Geometry check sheet. Reference: drawing and pictorial views, mm from the part's lowest x, y, z. A direction names the side the tool comes from. Round coordinates to 2 decimals unless told otherwise and drop trailing zeros. Loops run counter-clockwise (first coordinate to the right, second up) from the corner with the lowest first, then second, coordinate; pieces in that order, holes last. Notation, with made-up numbers: M -9,-7 L 40,-7 A9 cw 40,-1 Z; hole C 41.25,-34.75 d9. An arc over 180 degrees is marked long. One line per question, with ' | ' between items. Start each with the question number.
(1) Section check C-C (x = 2.25). Record the boundary of the cut face in (y, z) (1 decimal).
(2) Draft check along Z on the marked faces 1, 2 and 3. Enter one of: +Z half, -Z half, draft (parallel to the pull), parting line (faces both ways), or undercut.
(3) Section check B-B (z = 2.7). Record the boundary of the cut face in (x, y).
(4) Thickness scan on probe 1 along Z at (x, y) = (2.6, 3); probe 2 along Y at (x, z) = (4.6, 4.2); probe 3 along Y at (x, z) = (3.7, 3.35). Record the ranges inside material, lowest first. Write a range as [from, to].
(5) Section check D-D (y = 3.75). Record the boundary of the cut face in (x, z).
(6) Go/stop test with flat-tipped pins: P1, Ø1.5, axis at y = 4.5, z = 1.5, coming from the -X side (1 decimal); P2, Ø3, axis at y = 2, z = 2.5, coming from the +X side; P3, Ø1.2, axis at x = 2.5, z = 3, coming from the +Y side. Record where each tip stops, or that it passes through.
(7) Tool access check on the marked faces 4 and 5. Record the directions out of +Z, -Z, +X, -X, +Y, -Y that give a thin tool (end or side, any length) a straight path to the whole face; none if there is none.
(8) Section check A-A (y = 8). Record the boundary of the cut face in (x, z).
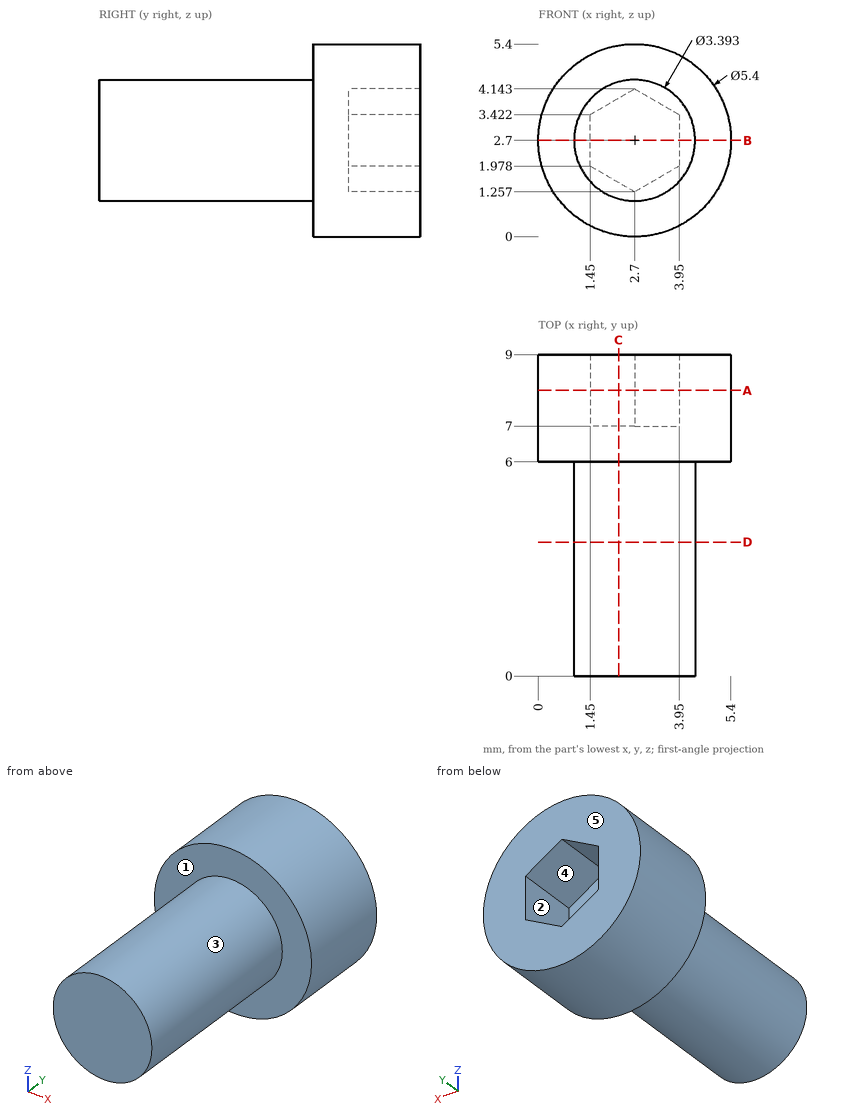
The answers:
1) outline: M 0,1.1 L 6,1.1 L 6,0 L 9,0 L 9,1.5 L 7,1.5 L 7,3.9 L 9,3.9 L 9,5.4 L 6,5.4 L 6,4.3 L 0,4.3 Z
2) face 1: draft | face 2: undercut | face 3: parting line
3) outline: M 0,6 L 1,6 L 1,0 L 4.4,0 L 4.4,6 L 5.4,6 L 5.4,9 L 3.95,9 L 3.95,7 L 1.45,7 L 1.45,9 L 0,9 Z
4) probe 1: [1.01, 4.39] | probe 2: [6, 9] | probe 3: [0, 7]
5) outline: C 2.7,2.7 d3.39
6) P1: x = 1.1 | P2: x = 4.4 | P3: y = 7
7) face 4: +Y | face 5: +Z, -Z, +X, -X, +Y
8) outline: C 2.7,2.7 d5.4; hole M 1.45,1.98 L 2.7,1.26 L 3.95,1.98 L 3.95,3.42 L 2.7,4.14 L 1.45,3.42 Z
